from build123d import *

# Parameters (mm, degrees)
BOSS_EXTRUDE1_DEPTH = 124
SKETCH2_R           = 44.45
CUT_EXTRUDE1_DEPTH  = 78
SKETCH3_R           = 28.575
CUT_EXTRUDE2_DEPTH  = 170
CUT_EXTRUDE3_DEPTH  = 13
CUT_EXTRUDE4_DEPTH  = 176.681530048
BOSS_EXTRUDE2_START = 33
BOSS_EXTRUDE2_DEPTH = 33


with BuildPart() as part:
    # Sketch1 → Boss-Extrude1 (new, symmetric)
    with BuildSketch(Plane(origin=(0, 0, 0), x_dir=(0, 0, -1), z_dir=(1, 0, 0))):
        with BuildLine():
            Line((0, 88), (0, -88))
            Line((0, -88), (-13, -88))
            Line((-13, -88), (-88, -44.698729811))
            Line((-88, -44.698729811), (-88, 0))
            ThreePointArc((-88, 0), (-62.225396744, 62.225396744), (0, 88))
        make_face()
    extrude(amount=BOSS_EXTRUDE1_DEPTH, both=True)

    # Sketch2 → Cut-Extrude1 (cut)
    with BuildSketch(Plane(origin=(124, 0, 0), x_dir=(0, 0, -1), z_dir=(1, 0, 0))):
        Circle(SKETCH2_R)
    extrude(amount=-CUT_EXTRUDE1_DEPTH, mode=Mode.SUBTRACT)

    # Sketch3 → Cut-Extrude2 (cut)
    with BuildSketch(Plane.ZY.offset(124)):
        Circle(SKETCH3_R)
    extrude(amount=-CUT_EXTRUDE2_DEPTH, mode=Mode.SUBTRACT)

    # Sketch4 → Cut-Extrude3 (cut)
    with BuildSketch(Plane(origin=(0, 0, 0), x_dir=(-1, 0, 0), z_dir=(0, 0, -1))):
        with BuildLine():
            Line((124, -73), (11, -73))
            ThreePointArc((11, -73), (0, -62), (11, -51))
            Line((11, -51), (124, -51))
            Line((124, -51), (124, -73))
        make_face()
    extrude(amount=-CUT_EXTRUDE3_DEPTH, mode=Mode.SUBTRACT)

    # Sketch5 → Cut-Extrude4 (cut, through all)
    with BuildSketch(Plane(origin=(0, 0, 0), x_dir=(1, 0, 0), z_dir=(0, 1, 0))):
        Polygon((-53, 0), (-86, 0), (-84.337715393, -19), (-54.662284607, -19), align=None)
    extrude(amount=CUT_EXTRUDE4_DEPTH, mode=Mode.SUBTRACT)

    # Sketch6 → Boss-Extrude2 (add)
    with BuildSketch(Plane(origin=(124, 0, 0), x_dir=(0, 0, -1), z_dir=(1, 0, 0)).offset(BOSS_EXTRUDE2_START)):
        with BuildLine():
            Line((-36.116548227, 80.247086827), (-14.946427946, 63.707176139))
            Line((-14.946427946, 63.707176139), (-65.430668922, -0.909705656))
            Line((-65.430668922, -0.909705656), (-86.600789204, 15.630205031))
            ThreePointArc((-86.600789204, 15.630205031), (-69.344946317, 54.178209829), (-36.116548227, 80.247086827))
        make_face()
    extrude(amount=-BOSS_EXTRUDE2_DEPTH)


solid = part.part
For this review, take the finished solid that the model builds, in its own axes (mm). A direction names the side the tool comes from. Round coordinates to 2 decimals unless told otherwise and drop trailing zeros. Order: outer loops, then holes, each group sorted by start corner. A loop starts at its lowest first (then second) coordinate and runs counter-clockwise, first axis right, second up. Notation, with made-up numbers: M 0.25,81.25 L 9.25,81.25 A24 cw 9.25,109.25 Z; hole C 30.5,36 d11. An arc over 180 degrees is marked long. Use a Markdown table: item, result. Add a question column.
Item 1: Mouldability with a two-part tool opening along Y and no side actions: class faces 1 (the flat face through (1.74, -66.65, 49.98)), 2 (the flat face through (46, 1, 32)), 3 (the flat face through (124, -18, 43)) as released by +Y, released by -Y, zero draft, split by the parting line, or undercut.
Item 2: To check wall thickness, follow line 1 along X through (y, z) = (2.5, 70.5); line 2 along Z through (x, y) = (-95, 1.5); line 3 along Y through (x, z) = (57.5, 38.5). State the ranges of each line that lie inside material, in increasing order.
Item 3: Add section A-A, the plane x = 31. Give the boundary of the cut face in (y, z) (3 decimals).
Item 4: Add section C-C, the plane x = -40. Give the boundary of the cut face in (y, z) (3 decimals).
Item 5: Tool access review of faces 4 (the flat face through (140.731, 7.244, 75.868)), 5 (the cylindrical face through (85.55, 0.98, 44.44)), 6 (the flat face through (-53.843, 54.205, 9.633)), 7 (the flat face through (-67, -51, 6)): name each direction out of +Z, -Z, +X, -X, +Y, -Y from which nothing blocks a thin tool from reaching the whole face with its end or side.
Item 6: Insertion check: pin 1 (1.5 mm diameter, centred on x = 51, z = 29.5, fed in from -Y); pin 2 (10 mm diameter, centred on x = -45.5, z = 73, fed in from +Y); pin 3 (24 mm diameter, centred on x = -81, y = -63, fed in from -Z); pin 4 (4 mm diameter, centred on x = -90, z = 9, fed in from +Y). Each pin has a flat end and moves straight along its axis. Give the tip position at first contact, or say it passes through.
Item 7: Add section B-B, the plane y = 55. Give the boundary of the cut face in (x, z).
Item 8: Add section D-D, the plane y = 33. Give the boundary of the cut face in (x, z), then the cut area to 3 significant figures.
Geometry results:
| question | item | result |
|---|---|---|
| 1 | face 1 | released by -Y |
| 1 | face 2 | undercut |
| 1 | face 3 | zero draft |
| 2 | line 1 | x = -124 to 124 |
| 2 | line 2 | z = 28.54 to 87.99 |
| 2 | line 3 | y = -73.28 to -22.22, 22.22 to 79.13 |
| 3 | outline | M -88,0 L -28.575,0 A28.575 cw 28.575,0 L 88,0 A88 ccw 0,88 L -44.699,88 L -88,13 Z |
| 4 | outline | M -88,0 L -73,0 L -73,13 L -51,13 L -51,0 L -28.575,0 A28.575 cw 28.575,0 L 88,0 A88 ccw 0,88 L -44.699,88 L -88,13 Z |
| 5 | face 4 | +Z, +X, -Y |
| 5 | face 5 | -Z, +X |
| 5 | face 6 | -Z, +Y |
| 5 | face 7 | -Z, -X |
| 6 | pin 1 | stops at y = -78.91 |
| 6 | pin 2 | stops at y = 55.86 |
| 6 | pin 3 | stops at z = 0 |
| 6 | pin 4 | stops at y = 87.72 |
| 7 | outline | M -124,0 L -86,0 L -84.34,19 L -54.66,19 L -53,0 L 124,0 L 124,21.75 L 157,21.75 L 157,68.69 L -124,68.69 Z |
| 8 | outline | M -124,0 L -86,0 L -84.34,19 L -54.66,19 L -53,0 L 46,0 L 46,29.78 L 124,29.78 L 124,38.94 L 157,38.94 L 157,81.58 L -124,81.58 Z |
| 8 | area | 18,700 mm² |
